from build123d import *

# Parameters (mm, degrees)
SKETCH1_W              = 12.319
SKETCH1_H              = 12.319
BOSS_EXTRUDE1_DEPTH    = 9.906
FILLET1_R              = 0.127
FILLET2_R              = 1.27
LPATTERN2_COUNT        = 2
LPATTERN2_PITCH        = 4.572
LPATTERN2_COUNT_DIR2   = 2
LPATTERN2_PITCH_DIR2   = 6.858
FILLET1_OF_LPATTERN2_R = 0.127
BOSS_EXTRUDE2_DEPTH    = 0.4826
FILLET3_R              = 0.254
LPATTERN5_COUNT        = 4
LPATTERN5_PITCH        = 2.54
FILLET3_OF_LPATTERN5_R = 0.254
MIRROR1_START          = -4.2926
MIRROR1_DEPTH          = 0.9652
MIRROR1_START_2        = -1.7526
MIRROR1_2_DEPTH        = 0.9652
MIRROR1_START_3        = 0.7874
MIRROR1_3_DEPTH        = 0.9652
MIRROR1_START_4        = 3.3274
MIRROR1_4_DEPTH        = 0.9652


# Read off the part's stored shape, not the designer's step: Mirror1
with BuildPart() as part:
    # Sketch1 → Boss-Extrude1 (new body)
    with BuildSketch(Plane(origin=(0, 0, 0), x_dir=(1, 0, 0), z_dir=(0, 1, 0))):
        Rectangle(SKETCH1_W, SKETCH1_H)
    extrude(amount=BOSS_EXTRUDE1_DEPTH)

    # Sketch3 → Revolve1 (revolve)
    with BuildSketch(Plane.XZ.offset(-8.509), mode=Mode.PRIVATE) as revolve1_sk:
        Polygon((-3.683, 6.1595), (-3.683, 9.8425), (-3.937, 9.8425), (-3.683, 12.7635), (-2.286, 12.7635), (-2.286, 6.1595), align=None)
    revolve1 = revolve(revolve1_sk.sketch.rotate(Axis((-2.286, 8.509, 12.7635), (0, 0, -1)), 180), axis=Axis((-2.286, 8.509, 12.7635), (0, 0, -1)))

    # Fillet1
    fillet1_edges = [part.edges().sort_by_distance(p)[0] for p in [
        (-3.937, 8.509, 9.8425),
        (-3.683, 8.509, 12.7635),
    ]]
    fillet(fillet1_edges, radius=FILLET1_R)

    # Fillet2
    fillet2_edges = [part.edges().sort_by_distance(p)[0] for p in [
        (6.1595, 4.953, 6.1595),
        (-6.1595, 4.953, 6.1595),
        (-6.1595, 4.953, -6.1595),
        (6.1595, 4.953, -6.1595),
    ]]
    fillet(fillet2_edges, radius=FILLET2_R)

    # LPattern2: Revolve1 2 × 2, 2 skipped
    with Locations(*[(i * LPATTERN2_PITCH, -j * LPATTERN2_PITCH_DIR2, 0) for i in range(LPATTERN2_COUNT) for j in range(LPATTERN2_COUNT_DIR2) if (i, j) not in ((0, 0), (0, 1), (1, 0))]):
        add(revolve1)

    # Fillet1 of LPattern2
    fillet1_of_lpattern2_edges = [part.edges().sort_by_distance(p)[0] for p in [
        (0.635, 1.651, 9.8425),
        (0.889, 1.651, 12.7635),
    ]]
    fillet(fillet1_of_lpattern2_edges, radius=FILLET1_OF_LPATTERN2_R)

    # Sketch5 → Boss-Extrude2 (add, symmetric)
    with BuildSketch(Plane(origin=(0, 0, 3.81), x_dir=(0, -1, 0), z_dir=(0, 0, 1))):
        Polygon((-3.81, 6.1595), (-3.81, 6.70408255), (0, 7.837886271), (0, 8.89), (-0.2794, 8.89), (-0.2794, 8.046249759), (-4.0894, 6.912446038), (-4.0894, 6.1595), align=None)
    boss_extrude2 = extrude(amount=BOSS_EXTRUDE2_DEPTH, both=True)

    # Fillet3
    fillet3_edges = [part.edges().sort_by_distance(p)[0] for p in [
        (6.70408255, 3.81, 3.81),
        (7.837886271, 0, 3.81),
        (8.046249759, 0.2794, 3.81),
        (6.912446038, 4.0894, 3.81),
    ]]
    fillet(fillet3_edges, radius=FILLET3_R)

    # LPattern5: Boss-Extrude2 ×4
    with Locations(*[(0, 0, -i * LPATTERN5_PITCH) for i in range(1, LPATTERN5_COUNT)]):
        add(boss_extrude2)

    # Fillet3 of LPattern5
    fillet3_of_lpattern5_edges = [part.edges().sort_by_distance(p)[0] for p in [
        (6.70408255, 3.81, 1.27),
        (7.837886271, 0, 1.27),
        (8.046249759, 0.2794, 1.27),
        (6.912446038, 4.0894, 1.27),
        (6.70408255, 3.81, -1.27),
        (7.837886271, 0, -1.27),
        (8.046249759, 0.2794, -1.27),
        (6.912446038, 4.0894, -1.27),
        (6.70408255, 3.81, -3.81),
        (7.837886271, 0, -3.81),
        (8.046249759, 0.2794, -3.81),
        (6.912446038, 4.0894, -3.81),
    ]]
    fillet(fillet3_of_lpattern5_edges, radius=FILLET3_OF_LPATTERN5_R)

    # Mirror1 outline → Mirror1 (add)
    with BuildSketch(Plane.XY.offset(MIRROR1_START)):
        with BuildLine():
            Line((-8.89, 0.2794), (-8.89, 0))
            Line((-8.89, 0), (-8.027307623, 0))
            ThreePointArc((-8.027307623, 0), (-7.875461582, 0.050385708), (-7.783858614, 0.181552915))
            Line((-7.783858614, 0.181552915), (-6.758110207, 3.628447085))
            ThreePointArc((-6.758110207, 3.628447085), (-6.666507239, 3.759614292), (-6.514661198, 3.81))
            Line((-6.514661198, 3.81), (-6.1595, 3.81))
            Line((-6.1595, 3.81), (-6.1595, 4.0894))
            Line((-6.1595, 4.0894), (-6.723024685, 4.0894))
            ThreePointArc((-6.723024685, 4.0894), (-6.874870727, 4.039014292), (-6.966473694, 3.907847085))
            Line((-6.966473694, 3.907847085), (-7.992222102, 0.460952915))
            ThreePointArc((-7.992222102, 0.460952915), (-8.08382507, 0.329785708), (-8.235671111, 0.2794))
            Line((-8.235671111, 0.2794), (-8.89, 0.2794))
        make_face()
    extrude(amount=MIRROR1_DEPTH)

    # Mirror1 2 outline → Mirror1 2 (add)
    with BuildSketch(Plane.XY.offset(MIRROR1_START_2)):
        with BuildLine():
            Line((-8.89, 0.2794), (-8.89, 0))
            Line((-8.89, 0), (-8.027307623, 0))
            ThreePointArc((-8.027307623, 0), (-7.875461582, 0.050385708), (-7.783858614, 0.181552915))
            Line((-7.783858614, 0.181552915), (-6.758110207, 3.628447085))
            ThreePointArc((-6.758110207, 3.628447085), (-6.666507239, 3.759614292), (-6.514661198, 3.81))
            Line((-6.514661198, 3.81), (-6.1595, 3.81))
            Line((-6.1595, 3.81), (-6.1595, 4.0894))
            Line((-6.1595, 4.0894), (-6.723024685, 4.0894))
            ThreePointArc((-6.723024685, 4.0894), (-6.874870727, 4.039014292), (-6.966473694, 3.907847085))
            Line((-6.966473694, 3.907847085), (-7.992222102, 0.460952915))
            ThreePointArc((-7.992222102, 0.460952915), (-8.08382507, 0.329785708), (-8.235671111, 0.2794))
            Line((-8.235671111, 0.2794), (-8.89, 0.2794))
        make_face()
    extrude(amount=MIRROR1_2_DEPTH)

    # Mirror1 3 outline → Mirror1 3 (add)
    with BuildSketch(Plane.XY.offset(MIRROR1_START_3)):
        with BuildLine():
            Line((-8.89, 0.2794), (-8.89, 0))
            Line((-8.89, 0), (-8.027307623, 0))
            ThreePointArc((-8.027307623, 0), (-7.875461582, 0.050385708), (-7.783858614, 0.181552915))
            Line((-7.783858614, 0.181552915), (-6.758110207, 3.628447085))
            ThreePointArc((-6.758110207, 3.628447085), (-6.666507239, 3.759614292), (-6.514661198, 3.81))
            Line((-6.514661198, 3.81), (-6.1595, 3.81))
            Line((-6.1595, 3.81), (-6.1595, 4.0894))
            Line((-6.1595, 4.0894), (-6.723024685, 4.0894))
            ThreePointArc((-6.723024685, 4.0894), (-6.874870727, 4.039014292), (-6.966473694, 3.907847085))
            Line((-6.966473694, 3.907847085), (-7.992222102, 0.460952915))
            ThreePointArc((-7.992222102, 0.460952915), (-8.08382507, 0.329785708), (-8.235671111, 0.2794))
            Line((-8.235671111, 0.2794), (-8.89, 0.2794))
        make_face()
    extrude(amount=MIRROR1_3_DEPTH)

    # Mirror1 4 outline → Mirror1 4 (add)
    with BuildSketch(Plane.XY.offset(MIRROR1_START_4)):
        with BuildLine():
            Line((-8.89, 0.2794), (-8.89, 0))
            Line((-8.89, 0), (-8.027307623, 0))
            ThreePointArc((-8.027307623, 0), (-7.875461582, 0.050385708), (-7.783858614, 0.181552915))
            Line((-7.783858614, 0.181552915), (-6.758110207, 3.628447085))
            ThreePointArc((-6.758110207, 3.628447085), (-6.666507239, 3.759614292), (-6.514661198, 3.81))
            Line((-6.514661198, 3.81), (-6.1595, 3.81))
            Line((-6.1595, 3.81), (-6.1595, 4.0894))
            Line((-6.1595, 4.0894), (-6.723024685, 4.0894))
            ThreePointArc((-6.723024685, 4.0894), (-6.874870727, 4.039014292), (-6.966473694, 3.907847085))
            Line((-6.966473694, 3.907847085), (-7.992222102, 0.460952915))
            ThreePointArc((-7.992222102, 0.460952915), (-8.08382507, 0.329785708), (-8.235671111, 0.2794))
            Line((-8.235671111, 0.2794), (-8.89, 0.2794))
        make_face()
    extrude(amount=MIRROR1_4_DEPTH)


solid = part.part
Verification items for the finished model (mm, model axes). A direction names the side the tool comes from. Coordinates: 2 decimals unless noted, no trailing zeros. Order: outer loops, then holes, each group sorted by start corner. A loop starts at its lowest first (then second) coordinate and runs counter-clockwise, first axis right, second up.
1. Set-up check for faces 1 (the face through (-7.28, 1.88, -3.82)), 2 (the face through (5.797, 5.022, -5.778)): record each of +Z, -Z, +X, -X, +Y, -Y from which the full face is reachable in a straight line by a thin tool's end or side.
Results found:
face 1: +Z, -Z, -Y
face 2: -Z, +X, +Y, -Y
2. Sectioned sample at C-C, the plane y = 6.5. Record the cut outline in (x, z), and give its area (3 significant figures).
Results found:
outline: (-6.16, -4.89) arc R1.27 ccw to (-4.89, -6.16) - (4.89, -6.16) arc R1.27 ccw to (6.16, -4.89) - (6.16, 4.89) arc R1.27 ccw to (4.89, 6.16) - (-4.89, 6.16) arc R1.27 ccw to (-6.16, 4.89) - close
area: 150 mm2
3. Sectioned sample at A-A, the plane z = 1.25. Record the cut outline in (x, y), and give its area (3 significant figures).
Results found:
outline: (-8.89, 0) - (-8.03, 0) arc R0.25 ccw to (-7.78, 0.18) - (-6.76, 3.63) arc R0.25 cw to (-6.51, 3.81) - (-6.16, 3.81) - (-6.16, 0) - (6.16, 0) - (6.16, 3.81) - (6.51, 3.81) arc R0.25 cw to (6.76, 3.63) - (7.78, 0.18) arc R0.25 ccw to (8.03, 0) - (8.89, 0) - (8.89, 0.28) - (8.24, 0.28) arc R0.25 cw to (7.99, 0.46) - (6.97, 3.91) arc R0.25 ccw to (6.72, 4.09) - (6.16, 4.09) - (6.16, 9.91) - (-6.16, 9.91) - (-6.16, 4.09) - (-6.72, 4.09) arc R0.25 ccw to (-6.97, 3.91) - (-7.99, 0.46) arc R0.25 cw to (-8.24, 0.28) - (-8.89, 0.28) - close
area: 125 mm2
4. Go/stop test with flat-tipped pins: pin 1 Ø1.4 at (x, y) = (7, 2.5) entering from +Z; pin 2 Ø1 at (y, z) = (8, -3) entering from +X; pin 3 Ø0.5 at (x, z) = (6.5, 1.5) entering from +Y. Record where each tip stops, or that it passes through.
Results found:
pin 1: stops at z = 4.29
pin 2: stops at x = 6.16
pin 3: stops at y = 4.09
5. Scan lines: line 1 (X direction, y = 2.75, z = 3.5); line 2 (Z direction, x = 2.75, y = 4); line 3 (Y direction, x = -6, z = 0.25). Record each from-to range of solid material in increasing order.
Results found:
line 1: x = -7.31 to -7.02, -6.16 to 6.16, 7.02 to 7.31
line 2: z = -6.16 to 6.16
line 3: y = 0 to 9.91
6. Sectioned sample at D-D, the plane z = 11.75. Record the cut outline in (x, y).
Results found:
outline: circle Ø2.97 at (-2.29, 8.51); circle Ø2.97 at (2.29, 1.65)
7. Sectioned sample at B-B, the plane x = -7.5. Record the cut outline in (y, z) (3 decimals).
Results found:
outline: (1.135, -4.293) - (2.115, -4.293) - (2.115, -3.327) - (1.135, -3.327) - close; (1.135, -1.753) - (2.115, -1.753) - (2.115, -0.787) - (1.135, -0.787) - close; (1.135, 0.787) - (2.115, 0.787) - (2.115, 1.753) - (1.135, 1.753) - close; (1.135, 3.327) - (2.115, 3.327) - (2.115, 4.293) - (1.135, 4.293) - close
